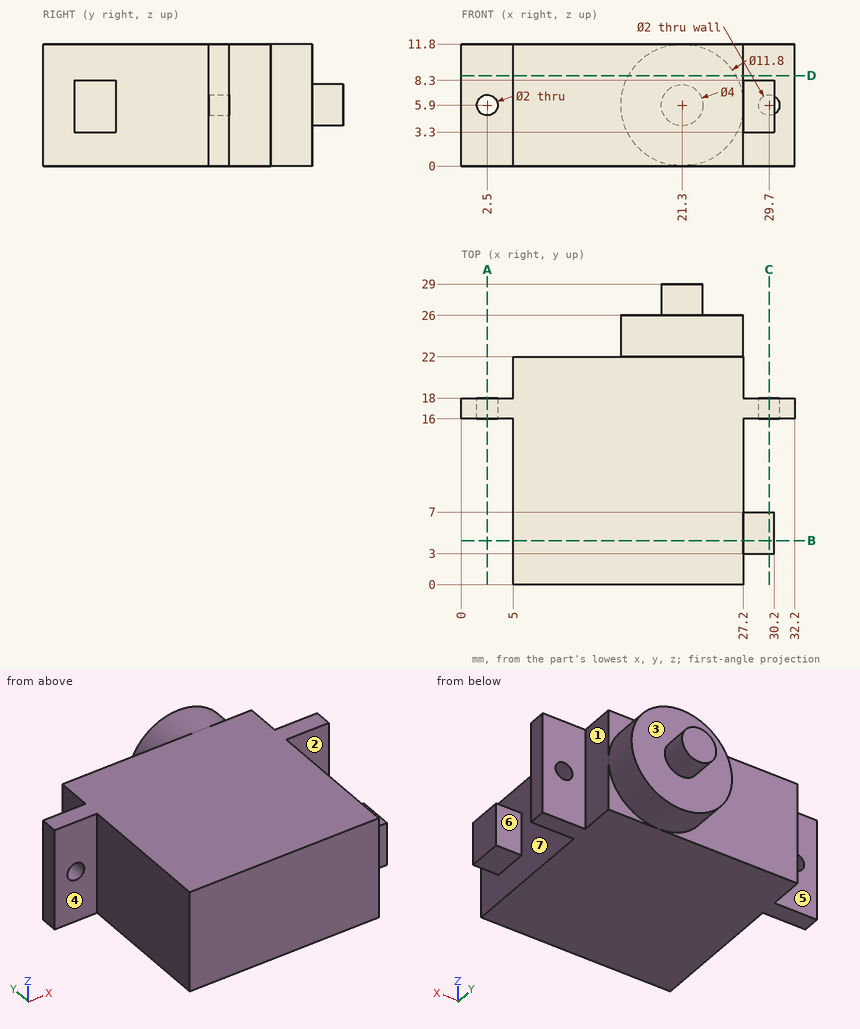
Print and shaded views of the part. All mm, measured from the part's lowest x, y and z. A direction names the side the tool comes from. Give positions to 0.01 mm unless a question says otherwise; leave off trailing zeros. Write each loop counter-clockwise with the first axis right and the second up, starting at its lowest first coordinate (ties: lowest second). Pieces come first, ordered by that corner, then holes. Notation, with made-up numbers: (86, 48.25) -> (142, 48.25) arc R21 ccw to (142, 83.25) -> close; hole circle Ø2 at (72.25, 36.25). An arc over 180 degrees is marked (long way). Write each question's results on one line, items separated by ' | '.
1. Two-plate mould, pull along Y, no slides. Class the marked faces 4, 5, 6 and 7: pulls with the +Y half, pulls with the -Y half, needs draft (parallel to the pull), parting line crosses it, or undercut.
Geometry check:
face 4: pulls with the -Y half | face 5: pulls with the +Y half | face 6: undercut | face 7: undercut
2. Cut at B-B, the plane y = 4.25. Write the cut outline in (x, z).
Geometry check:
outline: (5, 0) -> (27.2, 0) -> (27.2, 3.3) -> (30.2, 3.3) -> (30.2, 8.3) -> (27.2, 8.3) -> (27.2, 11.8) -> (5, 11.8) -> close
3. Wall check: probe 1 along Z at (x, y) = (2.5, 16.9); probe 2 along X at (y, z) = (17.2, 5.9); probe 3 along Y at (x, z) = (20.5, 2.75). Give the ranges that are in metal, low to high. Write a range as [from, to].
Geometry check:
probe 1: [0, 4.9], [6.9, 11.8] | probe 2: [0, 1.5], [3.5, 28.7], [30.7, 32.2] | probe 3: [0, 26]
4. Which spindle directions (+Z, -Z, +X, -X, +Y, -Y) get a long thin tool onto all of the face, cutting with end or side? Do the marked faces 1, 2 and 3. Say none if no direction does.
Geometry check:
face 1: +Z, -Z, +X, +Y | face 2: +Z, -Z, +X | face 3: +Y
5. Cut at A-A, the plane x = 2.5. Write the cut outline in (y, z).
Geometry check:
outline: (16, 0) -> (18, 0) -> (18, 4.9) -> (16, 4.9) -> close; (16, 6.9) -> (18, 6.9) -> (18, 11.8) -> (16, 11.8) -> close
6. Cut at C-C, the plane x = 29.7. Write the cut outline in (y, z), then the cut area to 3 significant figures.
Geometry check:
outline: (3, 3.3) -> (7, 3.3) -> (7, 8.3) -> (3, 8.3) -> close; (16, 0) -> (18, 0) -> (18, 4.9) -> (16, 4.9) -> close; (16, 6.9) -> (18, 6.9) -> (18, 11.8) -> (16, 11.8) -> close | area: 39.6 mm²
7. Drop flat-ended pins along their axis: P1, Ø0.9, axis at x = 28.5, z = 4.5, coming from the -Y side; P2, Ø6.5, axis at x = 25, z = 10, coming from the +Y side; P3, Ø1, axis at x = 10.5, z = 1.5, coming from the +Y side. Give the stop position or say it passes through.
Geometry check:
P1: y = 3 | P2: y = 26 | P3: y = 22
8. Cut at D-D, the plane z = 8.75. Write the cut outline in (x, y).
Geometry check:
outline: (0, 16) -> (5, 16) -> (5, 0) -> (27.2, 0) -> (27.2, 16) -> (32.2, 16) -> (32.2, 18) -> (27.2, 18) -> (27.2, 22) -> (26.47, 22) -> (26.47, 26) -> (16.13, 26) -> (16.13, 22) -> (5, 22) -> (5, 18) -> (0, 18) -> close
